Could you check a few things on this model? Use its own coordinates, in mm. Round coordinates to 2 decimals unless told otherwise and drop trailing zeros. Loops run counter-clockwise (first coordinate to the right, second up) from the corner with the lowest first, then second, coordinate; pieces in that order, holes last. Notation, with made-up numbers: (-20, 21) -> (15, 21) arc R13 ccw to (15, 39) -> close; hole circle Ø8 at (-27, 64.5). An arc over 180 degrees is marked (long way). One line per item, written item: value.
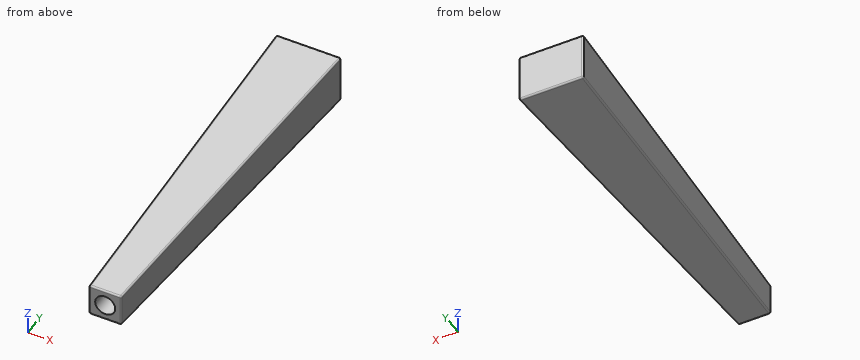
from build123d import *

# Parameters (mm, degrees)
F0_W      = 25.4
F0_H      = 19.05
F1_DEPTH  = 146.05
F4_DEPTH  = 25.4
F6_DEPTH  = 25.4
F8_DEPTH  = 12.7
F9_R      = 0.635
F10_R     = 3.937
F11_DEPTH = 31.75


with BuildPart() as f1:
    # F0 (on Front) → F1 (new body)
    with BuildSketch(Plane.XZ):
        Rectangle(F0_W, F0_H)
    extrude(amount=F1_DEPTH)

    # F3 (on face) → F4 (cut)
    with BuildSketch(Plane(origin=(-12.7, 0, 0), x_dir=(0, -1, 0), z_dir=(-1, 0, 0))):
        Polygon((146.05, 9.525), (0, 9.525), (146.05, 6.35), align=None)
    extrude(amount=-F4_DEPTH, mode=Mode.SUBTRACT)

    # F5 (on face) → F6 (cut)
    with BuildSketch(Plane(origin=(-12.7, 0, 0), x_dir=(0, -1, 0), z_dir=(-1, 0, 0))):
        Polygon((146.05, -6.35), (0, -9.525), (146.05, -9.525), align=None)
    extrude(amount=-F6_DEPTH, mode=Mode.SUBTRACT)

    # F7 (on Top) → F8 (cut, symmetric)
    with BuildSketch(Plane.XY):
        Polygon((-12.7, -146.05), (-6.35, -146.05), (-12.7, 0), align=None)
        Polygon((6.35, -146.05), (12.7, -146.05), (12.7, 0), align=None)
    extrude(amount=F8_DEPTH, both=True, mode=Mode.SUBTRACT)

    # F9
    f9_edges = [f1.edges().sort_by_distance(p)[0] for p in [
        (9.525, -73.025, 7.9375),
        (0, -146.05, 6.35),
        (6.35, -146.05, 0),
        (0, -146.05, -6.35),
        (-6.35, -146.05, 0),
        (-9.525, -73.025, 7.9375),
        (-9.525, -73.025, -7.9375),
        (12.7, 0, 0),
        (0, 0, 9.525),
        (-12.7, 0, 0),
        (0, 0, -9.525),
        (9.525, -73.025, -7.9375),
    ]]
    fillet(f9_edges, radius=F9_R)

    # F10 (on face) → F11 (cut)
    with BuildSketch(Plane.XZ.offset(146.05)):
        Circle(F10_R)
    extrude(amount=-F11_DEPTH, mode=Mode.SUBTRACT)


solid = f1.part
(1) If I drill on L1, parallel to Y at x = -3.5, z = -0.75; L2, parallel to Z at x = 0, y = -133; L3, parallel to Z at x = 0, y = -130, over which ranges is the centre line in solid material (lowest first)?
Recorded:
L1: -114.3 to 0
L2: -6.63 to -3.94, 3.94 to 6.63
L3: -6.7 to -3.94, 3.94 to 6.7
(2) If we section it at A-A, the plane z = 0: Please give me the cut outline in (x, y) (3 decimals).
Recorded:
outline: (-12.671, -0.663) -> (-6.376, -145.443) arc R0.635 ccw to (-5.742, -146.05) -> (-3.937, -146.05) -> (-3.937, -114.3) -> (3.937, -114.3) -> (3.937, -146.05) -> (5.742, -146.05) arc R0.635 ccw to (6.376, -145.443) -> (12.671, -0.663) arc R0.635 ccw to (12.037, 0) -> (-12.037, 0) arc R0.635 ccw to start
(3) I'm going to push flat-ended pins straight in: pin 1 Ø1 at (x, y) = (1.5, -51) entering from +Z; pin 2 Ø3 at (x, y) = (4, -129.5) entering from +Z; pin 3 Ø8 at (x, y) = (3, -103) entering from -Z. Where does each tip first touch, or does it pass through?
Recorded:
pin 1: z = 8.43
pin 2: z = 6.74
pin 3: z = -7.37
